Could you check a few things on this model? Use its own coordinates, in mm. A direction names the side the tool comes from. Give positions to 0.01 mm unless a question says otherwise; leave off trailing zeros. Write item = value, one per line. Start each with the question number.
```python
from build123d import *

# Parameters (mm, degrees)
SKETCH1_W           = 138.8
SKETCH1_H           = 47
BOSS_EXTRUDE1_DEPTH = 25
SKETCH2_W           = 10
SKETCH2_H           = 6.75
CUT_EXTRUDE1_DEPTH  = 5.15
SKETCH3_W           = 6.75
SKETCH3_H           = 3.95
CUT_EXTRUDE2_DEPTH  = 3
FILLET1_R           = 3
FILLET2_R           = 1
FILLET3_R           = 1


with BuildPart() as part:
    # Sketch1 → Boss-Extrude1 (new body)
    with BuildSketch(Plane(origin=(0, 0, 0), x_dir=(1, 0, 0), z_dir=(0, 1, 0))):
        Rectangle(SKETCH1_W, SKETCH1_H)
    extrude(amount=BOSS_EXTRUDE1_DEPTH)

    # Sketch2 → Cut-Extrude1 (cut)
    with BuildSketch(Plane(origin=(69.4, 0, 0), x_dir=(0, 0, -1), z_dir=(1, 0, 0))):
        with Locations((-13.5, 21.625)):
            Rectangle(SKETCH2_W, SKETCH2_H)
    extrude(amount=-CUT_EXTRUDE1_DEPTH, mode=Mode.SUBTRACT)

    # Sketch3 → Cut-Extrude2 (cut)
    with BuildSketch(Plane(origin=(69.4, 0, 0), x_dir=(0, 0, -1), z_dir=(1, 0, 0))):
        with Locations((14.925, 23.025)):
            Rectangle(SKETCH3_W, SKETCH3_H)
    extrude(amount=-CUT_EXTRUDE2_DEPTH, mode=Mode.SUBTRACT)

    # Fillet1
    fillet1_edges = [part.edges().sort_by_distance(p)[0] for p in [
        (-69.4, 12.5, 23.5),
        (-69.4, 12.5, -23.5),
        (69.4, 12.5, -23.5),
        (69.4, 12.5, 23.5),
    ]]
    fillet(fillet1_edges, radius=FILLET1_R)

    # Fillet2
    fillet2_edges = [part.edges().sort_by_distance(p)[0] for p in [
        (69.4, 25, -1.525),
        (69.4, 25, -19.4),
        (-69.4, 0, 0),
        (-69.4, 25, 0),
        (0, 0, 23.5),
        (0, 0, -23.5),
        (69.4, 0, 0),
        (-68.521320344, 0, 22.621320344),
        (68.521320344, 0, 22.621320344),
        (68.521320344, 0, -22.621320344),
        (-68.521320344, 0, -22.621320344),
        (0, 25, -23.5),
        (0, 25, 23.5),
        (69.4, 25, 19.5),
        (-68.521320344, 25, 22.621320344),
        (68.521320344, 25, 22.621320344),
        (68.521320344, 25, -22.621320344),
        (-68.521320344, 25, -22.621320344),
    ]]
    fillet(fillet2_edges, radius=FILLET2_R)

    # Fillet3
    fillet3_edges = [part.edges().sort_by_distance(p)[0] for p in [
        (64.25, 21.625, 18.5),
        (64.25, 21.625, 8.5),
        (66.4, 23.025, -11.55),
        (66.4, 23.025, -18.3),
    ]]
    fillet(fillet3_edges, radius=FILLET3_R)


solid = part.part
```
(1) On a 3-axis mill with a long thin cutter (end or side, diameter ignored), from which of +Z, -Z, +X, -X, +Y, -Y can I reach the whole of each face in a straight line? I mean faces 1 (the cylindrical face through (68.5, 12.66, 22.64)), 2 (the flat face through (67, 18.25, 14)). Say none if no direction works.
(2) If I drill on line 1 along X through (y, z) = (21.25, -12.5); line 2 along X through (y, z) = (22.25, 17), over which ranges is the centre line in solid material (lowest first)? Write a range as from..to.
(3) We'd pull the mould along Z, two halves only. Please class faces 3 (the flat face through (68, 21.05, -15)), 4 (the cylindrical face through (-68.54, 12.66, -22.6)), 5 (the flat face through (-1, 12, 23.5)): released by +Z, released by -Z, zero draft, split by the parting line, or undercut.
(4) I'm going to push flat-ended pins straight in: pin 1 (0.6 mm diameter, centred on x = 68.5, y = 22.5, fed in from +Z); pin 2 (1.2 mm diameter, centred on y = 23, z = -15.5, fed in from +X); pin 3 (1 mm diameter, centred on x = 68.5, y = 23, fed in from -Z). Where does each tip first touch, or does it pass through?
Answers below:
q1.face_1 = +Z, +X, +Y, -Y
q1.face_2 = +X, +Y
q2.line_1 = -69.4..66.4
q2.line_2 = -69.4..64.25
q3.face_3 = undercut
q3.face_4 = released by -Z
q3.face_5 = released by +Z
q4.pin_1 = 22.9
q4.pin_2 = 66.4
q4.pin_3 = -23.04
